Verification items for this drawing (mm, ordinates from the low corner). Round coordinates to 2 decimals unless told otherwise and drop trailing zeros. Loops run counter-clockwise (first coordinate to the right, second up) from the corner with the lowest first, then second, coordinate; pieces in that order, holes last. Notation, with made-up numbers: (40.5, -23.75) -> (86.5, -23.75) arc R17 ccw to (86.5, -17.75) -> close; hole circle Ø9 at (65, 66). An arc over 180 degrees is marked (long way). One line per question, with ' | ' between items.
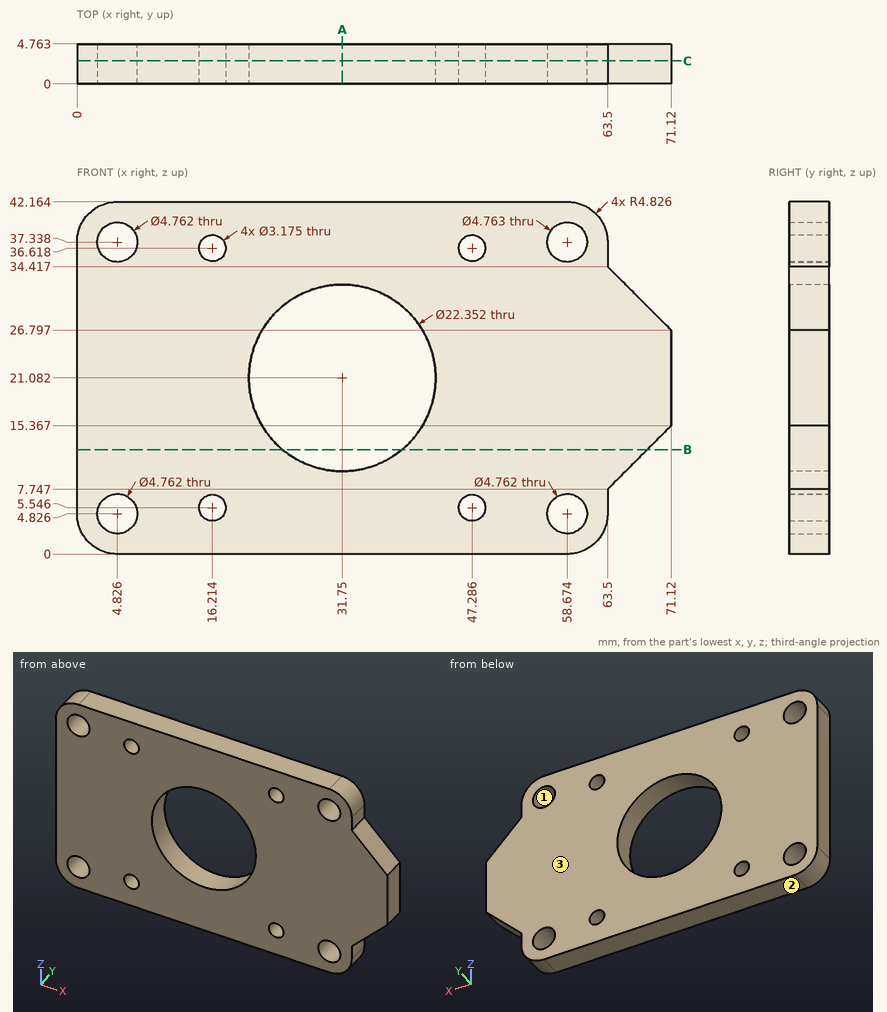
(1) Sectioned sample at A-A, the plane x = 31.75. Record the cut outline in (y, z) (1 decimal).
Answer:
outline: (0, 0) -> (4.8, 0) -> (4.8, 9.9) -> (0, 9.9) -> close; (0, 32.3) -> (4.8, 32.3) -> (4.8, 42.2) -> (0, 42.2) -> close
(2) Sectioned sample at C-C, the plane y = 2.75. Count the separate pieces of the cut face and the enclosed holes in it, and give its area (3 significant figures).
Answer:
separate pieces: 1 | enclosed holes: 9 | area: 2,310 mm2
(3) Go/stop test with a flat-tipped pin: pin 1 (1.5 mm diameter, centred on y = 1.5, z = 6.5, fed in from +X). Record where the tip stops, or that it passes through.
Answer:
pin 1: stops at x = 63.5
(4) Mould release check, pull along Z, two halves, no side actions. Record for the marked faces 1, 2 and 3: +Z half, -Z half, draft (parallel to the pull), parting line (faces both ways), or undercut.
Answer:
face 1: undercut | face 2: -Z half | face 3: draft
(5) Sectioned sample at B-B, the plane z = 12.5. Record the cut outline in (x, y), and give its area (3 significant figures).
Answer:
outline: (0, 0) -> (24.59, 0) -> (24.59, 4.76) -> (0, 4.76) -> close; (38.91, 0) -> (68.25, 0) -> (68.25, 4.76) -> (38.91, 4.76) -> close | area: 257 mm2
(6) Scan lines: probe 1 along Z at (x, y) = (3, 1.7) (1 decimal); probe 2 along X at (y, z) = (3.15, 39) (1 decimal); probe 3 along X at (y, z) = (1.5, 6.5) (1 decimal). Record each from-to range of solid material in increasing order.
Answer:
probe 1: z = 0.4 to 3.3, 6.4 to 35.8, 38.9 to 41.8 | probe 2: x = 0.3 to 3.1, 6.5 to 57, 60.4 to 63.2 | probe 3: x = 0 to 3.1, 6.5 to 14.9, 17.5 to 46, 48.6 to 57, 60.4 to 63.5
